Here's how the part is built. I have some questions about the finished solid (model axes, mm). A direction names the side the tool comes from. Round coordinates to 2 decimals unless told otherwise and drop trailing zeros. Order: outer loops, then holes, each group sorted by start corner. A loop starts at its lowest first (then second) coordinate and runs counter-clockwise, first axis right, second up. Notation, with made-up numbers: (15, -14.5) - (59, -14.5) arc R17 cw to (59, -2.5) - close; hole circle Ø7 at (36, 19). An arc over 180 degrees is marked (long way). Answer as a JSON object with one key per item and string values.
```python
from build123d import *

# Parameters (mm, degrees)
SKETCH1_W                             = 70
SKETCH1_H                             = 70
F_125_IN_SHEET_DEPTH                  = 3.175
FILLET1_R                             = 5
FILLET2_R                             = 20
F_5_0_REAMED_OVER_FOR_SHOULDER_BOLT_D = 5
M3X0_5_TAPPED_HOLE1_REACH             = 80.327
M3X0_5_TAPPED_HOLE1_BORE_R            = 1.25


with BuildPart() as part:
    # Sketch1 → .125 in sheet (new, symmetric)
    with BuildSketch(Plane.XY):
        Rectangle(SKETCH1_W, SKETCH1_H)
        with BuildLine():
            Line((-15.75784645, 25), (15.75784645, 25))
            ThreePointArc((15.75784645, 25), (17.67766953, 17.67766953), (25, 15.75784645))
            Line((25, 15.75784645), (25, -15.75784645))
            ThreePointArc((25, -15.75784645), (17.67766953, -17.67766953), (15.75784645, -25))
            Line((15.75784645, -25), (-15.75784645, -25))
            ThreePointArc((-15.75784645, -25), (-17.67766953, -17.67766953), (-25, -15.75784645))
            Line((-25, -15.75784645), (-25, 15.75784645))
            ThreePointArc((-25, 15.75784645), (-17.67766953, 17.67766953), (-15.75784645, 25))
        make_face(mode=Mode.SUBTRACT)
    extrude(amount=F_125_IN_SHEET_DEPTH, both=True)

    # Fillet1
    fillet1_edges = [part.edges().sort_by_distance(p)[0] for p in [
        (25, 15.75784645, 0),
        (15.75784645, 25, 0),
        (-15.75784645, 25, 0),
        (-25, 15.75784645, 0),
        (-25, -15.75784645, 0),
        (-15.75784645, -25, 0),
        (15.75784645, -25, 0),
        (25, -15.75784645, 0),
    ]]
    fillet(fillet1_edges, radius=FILLET1_R)

    # Fillet2
    fillet2_edges = [part.edges().sort_by_distance(p)[0] for p in [
        (-35, -35, 0),
        (-35, 35, 0),
        (35, 35, 0),
        (35, -35, 0),
    ]]
    fillet(fillet2_edges, radius=FILLET2_R)

    # Ø5.0 Reamed over for shoulder bolt (through all)
    with Locations(Plane(origin=(-38.607659372, 4.370839302, 3.175), x_dir=(1, 0, 0), z_dir=(0, 0, 1))):
        with Locations((15.626688983, 18.610131087), (61.58862976, 18.610131087), (61.58862976, -27.35180969), (15.626688983, -27.35180969)):
            Hole(F_5_0_REAMED_OVER_FOR_SHOULDER_BOLT_D / 2)

    # M3x0.5 Tapped Hole1 bore → M3x0.5 Tapped Hole1 (cut, up to next)
    with BuildSketch(Plane(origin=(0, 35, 0), x_dir=(1, 0, 0), z_dir=(0, 1, 0)), mode=Mode.PRIVATE) as m3x0_5_tapped_hole1_sk1:
        with Locations((-12.5, 0)):
            Circle(M3X0_5_TAPPED_HOLE1_BORE_R)
    m3x0_5_tapped_hole1_tool1 = extrude(m3x0_5_tapped_hole1_sk1.sketch, amount=-M3X0_5_TAPPED_HOLE1_REACH, mode=Mode.PRIVATE) & part.part
    # M3x0.5 Tapped Hole1 bore → M3x0.5 Tapped Hole1 (cut, up to next)
    with BuildSketch(Plane(origin=(0, 35, 0), x_dir=(1, 0, 0), z_dir=(0, 1, 0)), mode=Mode.PRIVATE) as m3x0_5_tapped_hole1_sk2:
        with Locations((12.5, 0)):
            Circle(M3X0_5_TAPPED_HOLE1_BORE_R)
    m3x0_5_tapped_hole1_tool2 = extrude(m3x0_5_tapped_hole1_sk2.sketch, amount=-M3X0_5_TAPPED_HOLE1_REACH, mode=Mode.PRIVATE) & part.part
    m3x0_5_tapped_hole1_1 = m3x0_5_tapped_hole1_tool1.solids().sort_by_distance((-12.5, 35, 0))[0]
    add(m3x0_5_tapped_hole1_1, mode=Mode.SUBTRACT)
    m3x0_5_tapped_hole1_2 = m3x0_5_tapped_hole1_tool2.solids().sort_by_distance((12.5, 35, 0))[0]
    add(m3x0_5_tapped_hole1_2, mode=Mode.SUBTRACT)
    m3x0_5_tapped_hole1 = m3x0_5_tapped_hole1_1 + m3x0_5_tapped_hole1_2  # M3x0.5 Tapped Hole1 as one shape, for the pattern or mirror that repeats it

    # Mirror1: M3x0.5 Tapped Hole1 across plane
    add(m3x0_5_tapped_hole1.mirror(Plane.ZX), mode=Mode.SUBTRACT)


solid = part.part
```
1. Thinking about a two-plate mould opening in Z: for faces 3 (the face through (-13.75, 29.6, -0.05)), 4 (the face through (-22.44, -25.42, -0.04)), 5 (the face through (-24, 16, 3.175)), which applies, pulls with the +Z half, pulls with the -Z half, needs draft (parallel to the pull), parting line crosses it, or undercut?
Responses:
{"face 3": "undercut", "face 4": "needs draft", "face 5": "pulls with the +Z half"}
2. Imagine slicing it at D-D (x = -26.5). List the corners of the cut face in (y, z) for me (3 decimals).
Responses:
{"outline": "(-31.363, -3.175) - (31.363, -3.175) - (31.363, 3.175) - (-31.363, 3.175) - close"}
3. Imagine slicing it at B-B (z = 0). Give the number of separate pieces and of enclosed holes in the cut face, plus the area to 3 significant figures.
Responses:
{"separate pieces": "4", "enclosed holes": "4", "area": "2,220 mm2"}
4. For P1, Ø1, axis at y = 17, z = 2, coming from the +X side; P2, Ø2, axis at x = -12.5, z = 0, coming from the -Y side; P3, Ø2, axis at x = 25, z = 0.5, coming from the +Y side, each with a flat end and sliding along its axis, tell me the tip position at first contact or that it passes through.
Responses:
{"P1": "x = 34.94", "P2": "through", "P3": "y = 32.86"}
5. For faces 1 (the face through (-13.89, 23.963, 0.044)), 2 (the face through (-13.75, -29.6, -0.05)), which set-ups out of +Z, -Z, +X, -X, +Y, -Y let a thin tool reach every point of the face, with its end or its side?
Responses:
{"face 1": "+Z, -Z", "face 2": "+Y, -Y"}
6. Imagine slicing it at A-A (x = -6). List the corners of the cut face in (y, z) for me (3 decimals), plus the area to 3 significant figures.
Responses:
{"outline": "(-35, -3.175) - (-25, -3.175) - (-25, 3.175) - (-35, 3.175) - close; (25, -3.175) - (35, -3.175) - (35, 3.175) - (25, 3.175) - close", "area": "127 mm2"}
7. Imagine slicing it at C-C (x = -17.5). List the corners of the cut face in (y, z) for me (1 decimal).
Responses:
{"outline": "(-34.8, -3.2) - (-17.9, -3.2) - (-17.9, 3.2) - (-34.8, 3.2) - close; (17.9, -3.2) - (34.8, -3.2) - (34.8, 3.2) - (17.9, 3.2) - close"}
8. If I drill on L1, parallel to Y at x = 5, z = -2.5; L2, parallel to X at y = 22.5, z = 1.5, over which ranges is the centre line in solid material (lowest first)? Write a range as [from, to].
Responses:
{"L1": "[-35, -25], [25, 35]", "L2": "[-33.54, -25.43], [-20.53, -15.17], [15.17, 20.53], [25.43, 33.54]"}
